Autodesk Inventor part; units mm, degrees
ref_plane "YZ Plane" through (0, 0, 0) normal (1, 0, 0) x (0, 1, 0)
ref_plane "XZ Plane" through (0, 0, 0) normal (0, 1, 0) x (-1, 0, 0)
ref_plane "XY Plane" through (0, 0, 0) normal (0, 0, 1) x (1, 0, 0)
sketch "Sketch1" plane through (0, 0, 0) normal (0, 1, 0) x (-1, 0, 0)
  line L0 (0, 0) -> (50.8, 0)
  line L1 (50.8, 0) -> (50.8, 28.575)
  line L2 (50.8, 28.575) -> (0, 28.575)
  line L3 (0, 28.575) -> (0, 0)
  line L4 (0, 28.575) -> (50.8, 28.575)
  line L5 (50.8, 28.575) -> (50.8, 25.4)
  line L6 (47.625, 25.4) -> (3.175, 25.4)
  line L7 (0, 25.4) -> (0, 28.575)
  line L8 (47.625, 25.4) -> (47.625, 0)
  line L9 (47.625, 0) -> (50.8, 0)
  line L10 (50.8, 0) -> (50.8, 25.4)
  line L11 (0, 0) -> (3.175, 0)
  line L12 (3.175, 0) -> (3.175, 25.4)
  line L13 (0, 25.4) -> (0, 0)
  line L14 (25.4, 0) -> (27.94, 0)
  line L15 (25.4, 0) -> (22.86, 0)
  line L16 (22.86, 0) -> (27.94, 0)
  line L17 (27.94, 0) -> (27.94, 17.78)
  line L18 (22.86, 17.78) -> (22.86, 0)
  arc A0 (27.94, 17.78) -> (22.86, 17.78) centre (25.4, 17.78) ccw
  line L19 (3.175, 0) -> (6.985, 0)
  circle A1 centre (6.985, 6.477) radius 1.524
  line L20 (47.625, 0) -> (43.815, 0)
  circle A2 centre (43.815, 6.477) radius 1.524
  dimension "d0" = 50.8
  dimension "d1" = 28.575
  dimension "d2" = 3.175
  dimension "d3" = 3.175
  dimension "d4" = 3.175
  dimension "d5" = 2.54
  dimension "d6" = 2.54
  dimension "d11" = 3.048
  dimension "d12" = 3.81
extrude "Extrusion1" add sketch "Sketch1" along normal blind 3.175 contours L3 L2 L1 L0 L8 L6 L12 | L12 L6 L8 L0 L17 A0 L18
sketch "Sketch2" plane through (0, 3.175, 0) normal (0, 1, 0) x (1, 0, 0)
  line L0 (-27.94, 0) -> (-50.8, 0)
  line L1 (-50.8, 0) -> (-50.8, -28.575)
  line L2 (0, -28.575) -> (0, 0)
  line L3 (0, -28.575) -> (-50.8, -28.575)
  line L4 (-50.8, -28.575) -> (-50.8, -25.4)
  line L5 (-47.625, -25.4) -> (-3.175, -25.4)
  line L6 (0, -25.4) -> (0, -28.575)
  line L7 (-47.625, -25.4) -> (-47.625, 0)
  line L8 (-47.625, 0) -> (-50.8, 0)
  line L9 (-50.8, 0) -> (-50.8, -25.4)
  line L10 (0, 0) -> (-3.175, 0)
  line L11 (-3.175, 0) -> (-3.175, -25.4)
  line L12 (0, -25.4) -> (0, 0)
  dimension "d15" = 3.175
  dimension "d16" = 3.175
  dimension "d17" = 3.175
extrude "Extrusion2" add sketch "Sketch2" along normal blind 15.24
sketch "Sketch3" plane through (-3.175, 3.175, 25.4) normal (0, 0, -1) x (-1, 0, 0)
  line L0 (44.45, 0) -> (44.45, 15.24)
  line L1 (0, 15.24) -> (44.45, 15.24)
  line L2 (44.45, 15.24) -> (44.45, 12.065)
  line L3 (44.45, 12.065) -> (0, 12.065)
  line L4 (0, 12.065) -> (0, 15.24)
  point P0 (-3.175, -3.175)
  dimension "d20" = 3.175
extrude "Extrusion3" add sketch "Sketch3" along normal blind 13.97
properties part number "IR Cover"
Input: part model. Units: mm. Frame: model coordinates. A direction names the side the tool comes from. Round coordinates to 2 decimals unless told otherwise and drop trailing zeros. Loops run counter-clockwise (first coordinate to the right, second up) from the corner with the lowest first, then second, coordinate; pieces in that order, holes last.
1) Section query A-A on z = 10. Return the cut outline in (x, y) (3 decimals).
Ans:
outline: (-50.8, 0) - (-27.94, 0) - (-27.94, 3.175) - (-47.625, 3.175) - (-47.625, 18.415) - (-50.8, 18.415) - close; (-22.86, 0) - (0, 0) - (0, 18.415) - (-3.175, 18.415) - (-3.175, 3.175) - (-22.86, 3.175) - close
2) Section query D-D on x = -43. Return the cut outline in (y, z) (3 decimals), plus the area to 3 significant figures.
Ans:
outline: (0, 0) - (3.175, 0) - (3.175, 5.189) - (0, 5.189) - close; (0, 7.765) - (3.175, 7.765) - (3.175, 25.4) - (15.24, 25.4) - (15.24, 11.43) - (18.415, 11.43) - (18.415, 28.575) - (0, 28.575) - close
area: 175 mm2
3) Section query B-B on x = -25.4. Return the cut outline in (y, z) (3 decimals).
Ans:
outline: (0, 20.32) - (3.175, 20.32) - (3.175, 25.4) - (15.24, 25.4) - (15.24, 11.43) - (18.415, 11.43) - (18.415, 28.575) - (0, 28.575) - close
4) Section query C-C on y = 10.25. Return the cut outline in (x, z) (3 decimals).
Ans:
outline: (-50.8, 0) - (-47.625, 0) - (-47.625, 25.4) - (-3.175, 25.4) - (-3.175, 0) - (0, 0) - (0, 28.575) - (-50.8, 28.575) - close
5) Material intervals for line 1 (X direction, y = 2.25, z = 3.5); line 2 (X direction, y = 14.25, z = 21.5) (3 decimals); line 3 (Y direction, x = -15.5, z = 20.5) (3 decimals), sorted ascending.
Ans:
line 1: x = -50.8 to -27.94, -22.86 to 0
line 2: x = -50.8 to -47.625, -3.175 to 0
line 3: y = 0 to 3.175, 15.24 to 18.415
6) Pin query (flat end, axial travel): pin 1 (5 mm diameter, centred on x = -43.815, z = 6.477, fed in from +Y) (3 decimals); pin 2 (2.5 mm diameter, centred on x = -23.5, y = 17.5, fed in from -Z); pin 3 (3.5 mm diameter, centred on x = -34, y = 10.5, fed in from -Z). Return the tip coordinate at first contact, or that it passes through.
Ans:
pin 1: stops at y = 3.175
pin 2: stops at z = 11.43
pin 3: stops at z = 25.4
7) Pull-direction query (Y, two-part tool) for faces 1 (the cylindrical face through (-42.292, 1.565, 6.41)), 2 (the flat face through (-26, 18.415, 20)), 3 (the flat face through (-3.175, 11, 13)), 4 (the flat face through (-31, 0, 14)); classes: released by +Y, released by -Y, zero draft, split by the parting line, or undercut.
Ans:
face 1: zero draft
face 2: released by +Y
face 3: undercut
face 4: released by -Y
8) Set-up query: faces 5 (the flat face through (-26, 15.24, 19)), 6 (the flat face through (-27.94, 2, 9)), 7 (the flat face through (-25, 17, 11.43)). Return all of +Z, -Z, +X, -X, +Y, -Y with unobstructed straight access to the full face (end or side cutting, diameter ignored); none if empty.
Ans:
face 5: -Z
face 6: -Z, -Y
face 7: -Z, +Y
